Input: part model. Units: mm. Frame: model coordinates. Round coordinates to 2 decimals unless told otherwise and drop trailing zeros. Order: outer loops, then holes, each group sorted by start corner. A loop starts at its lowest first (then second) coordinate and runs counter-clockwise, first axis right, second up. Notation, with made-up numbers: (-30.5, 74.5) -> (23.5, 74.5) arc R13 cw to (23.5, 81.5) -> close; hole circle Ø5 at (28, 42.25). An arc over 180 degrees is marked (long way). Use a Markdown table: item, result.
from build123d import *

# Parameters (mm, degrees)
SKETCH_1_W      = 360
SKETCH_1_H      = 20
SKETCH_1_R      = 7
EXTRUDE_1_DEPTH = 10
FILLET_1_R      = 10


with BuildPart() as part:
    # 草图1 → 凸台-拉伸1 (new body)
    with BuildSketch(Plane.XY):
        Rectangle(SKETCH_1_W, SKETCH_1_H)
        with Locations((-170, 0)):
            Circle(SKETCH_1_R, mode=Mode.SUBTRACT)
        with Locations((170, 0)):
            Circle(SKETCH_1_R, mode=Mode.SUBTRACT)
    extrude(amount=EXTRUDE_1_DEPTH)

    # 圆角1
    fillet_1_edges = [part.edges().sort_by_distance(p)[0] for p in [
        (180, 10, 5),
        (180, -10, 5),
        (-180, -10, 5),
        (-180, 10, 5),
    ]]
    fillet(fillet_1_edges, radius=FILLET_1_R - 0.0001)  # a hair under: the kernel refuses the full size


solid = part.part
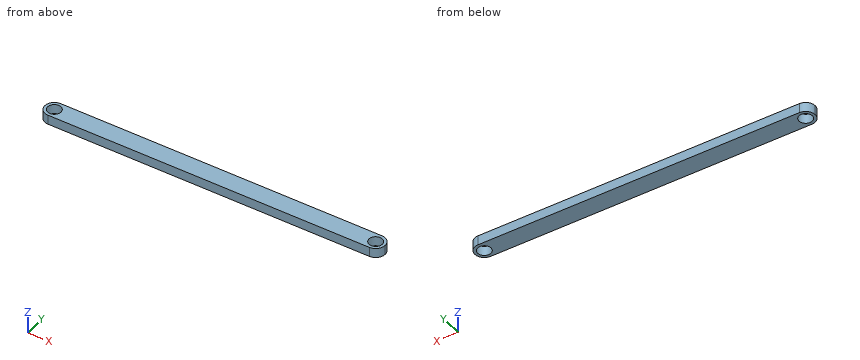
1) Pin query (flat end, axial travel): pin 1 Ø3 at (x, y) = (52.5, 0) entering from -Z. Return the tip coordinate at first contact, or that it passes through.
Results found:
| item | result |
|---|---|
| pin 1 | stops at z = 0 |
2) Cut plane A-A on y = 3.5. Return loops of the section in (x, z), and give its area (3 significant figures).
Results found:
| item | result |
|---|---|
| outline | (-179.37, 0) -> (-176.06, 0) -> (-176.06, 10) -> (-179.37, 10) -> close; (-163.94, 0) -> (163.94, 0) -> (163.94, 10) -> (-163.94, 10) -> close; (176.06, 0) -> (179.37, 0) -> (179.37, 10) -> (176.06, 10) -> close |
| area | 3,340 mm² |
3) Cut plane B-B on z = 1.75. Count the separate pieces of the cut face and the enclosed holes in it, and give its area (3 significant figures).
Results found:
| item | result |
|---|---|
| separate pieces | 1 |
| enclosed holes | 2 |
| area | 6,810 mm² |
4) Line query: L1, parallel to X at y = 0.25, z = 3.25; L2, parallel to Y at x = -170, z = 4; L3, parallel to X at y = 1.5, z = 0.5. Output: solid intervals per line, ascending. Write a range as [from, to].
Results found:
| item | result |
|---|---|
| L1 | x = [-180, -177], [-163, 163], [177, 180] |
| L2 | y = [-10, -7], [7, 10] |
| L3 | x = [-179.89, -176.84], [-163.16, 163.16], [176.84, 179.89] |
